Check sheet for the modelled part. Datum: model origin and axes. Units: mm. Face numbers are marked on the shaded views. A direction names the side the tool comes from. Round coordinates to 2 decimals unless told otherwise and drop trailing zeros. Write each loop counter-clockwise with the first axis right and the second up, starting at its lowest first coordinate (ties: lowest second). Pieces come first, ordered by that corner, then holes. Notation, with made-up numbers: (33.25, 46.25) -> (63.25, 46.25) arc R8 cw to (63.25, 52.25) -> close; hole circle Ø1 at (33, -17.5). An arc over 180 degrees is marked (long way). Write item = value, one per line.
from build123d import *

# Parameters (mm, degrees)
SKETCH1_W              = 165.1
SKETCH1_H              = 47.498
BOSS_EXTRUDE1_DEPTH    = 22.098
CUT_EXTRUDE1_DEPTH     = 18.249011
F_10_32_TAPPED_HOLE1_D = 4.0386


with BuildPart() as part:
    # Sketch1 → Boss-Extrude1 (new body)
    with BuildSketch(Plane(origin=(0, 0, 0), x_dir=(0, 0, -1), z_dir=(1, 0, 0))):
        Rectangle(SKETCH1_W, SKETCH1_H)
        with BuildLine():
            Line((-67.5752522, 2.5527), (67.5752522, 2.5527))
            ThreePointArc((67.5752522, 2.5527), (70.1279522, 0), (67.5752522, -2.5527))
            Line((67.5752522, -2.5527), (-67.5752522, -2.5527))
            ThreePointArc((-67.5752522, -2.5527), (-70.1279522, 0), (-67.5752522, 2.5527))
        make_face(mode=Mode.SUBTRACT)
    extrude(amount=BOSS_EXTRUDE1_DEPTH)

    # Sketch2 → Cut-Extrude1 (cut)
    with BuildSketch(Plane(origin=(22.098, 0, 0), x_dir=(0, 0, -1), z_dir=(1, 0, 0))):
        with BuildLine():
            Line((-67.5752522, 6.4797559), (67.5752522, 6.4797559))
            ThreePointArc((67.5752522, 6.4797559), (74.0550081, 0), (67.5752522, -6.4797559))
            Line((67.5752522, -6.4797559), (-67.5752522, -6.4797559))
            ThreePointArc((-67.5752522, -6.4797559), (-74.0550081, 0), (-67.5752522, 6.4797559))
        make_face()
    extrude(amount=-CUT_EXTRUDE1_DEPTH, mode=Mode.SUBTRACT)

    # #10-32 Tapped Hole1 (through all)
    with Locations(Plane(origin=(22.098, 0, 0), x_dir=(0, 0, -1), z_dir=(1, 0, 0))):
        with Locations((-76.2, 17.399), (-76.2, -17.399), (0, -17.399), (76.2, -17.399), (76.2, 17.399), (0, 17.399)):
            Hole(F_10_32_TAPPED_HOLE1_D / 2)


solid = part.part
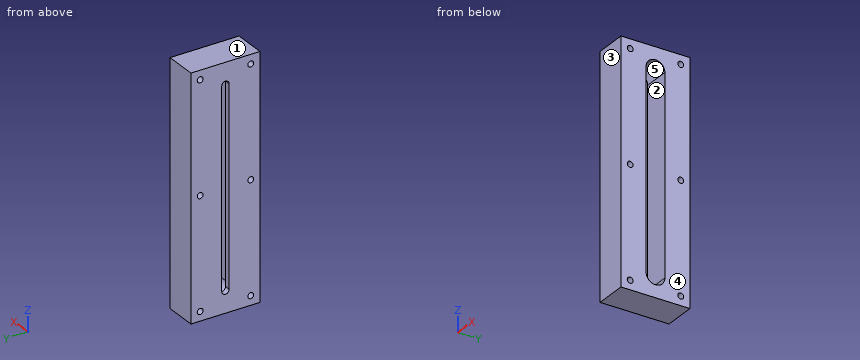
(1) Sectioned sample at C-C on y = 0.5. Enter the section's corners in (x, z).
Worked answers:
outline = (0, -82.55) -> (22.1, -82.55) -> (22.1, -74.04) -> (3.85, -74.04) -> (3.85, -70.08) -> (0, -70.08) -> close; (0, 70.08) -> (3.85, 70.08) -> (3.85, 74.04) -> (22.1, 74.04) -> (22.1, 82.55) -> (0, 82.55) -> close
(2) Sectioned sample at D-D on z = 76.2. Enter the section's corners in (x, y), then the cut area to 3 significant figures.
Worked answers:
outline = (0, -23.75) -> (22.1, -23.75) -> (22.1, -19.42) -> (0, -19.42) -> close; (0, -15.38) -> (22.1, -15.38) -> (22.1, 15.38) -> (0, 15.38) -> close; (0, 19.42) -> (22.1, 19.42) -> (22.1, 23.75) -> (0, 23.75) -> close
area = 871 mm²
(3) Sectioned sample at A-A on z = 0. Enter the section's corners in (x, y), then the cut area to 3 significant figures.
Worked answers:
outline = (0, -23.75) -> (22.1, -23.75) -> (22.1, -19.42) -> (0, -19.42) -> close; (0, -15.38) -> (22.1, -15.38) -> (22.1, -6.48) -> (3.85, -6.48) -> (3.85, -2.55) -> (0, -2.55) -> close; (0, 2.55) -> (3.85, 2.55) -> (3.85, 6.48) -> (22.1, 6.48) -> (22.1, 15.38) -> (0, 15.38) -> close; (0, 19.42) -> (22.1, 19.42) -> (22.1, 23.75) -> (0, 23.75) -> close
area = 615 mm²
(4) Go/stop test with flat-tipped pins: P1, Ø2.5, axis at y = -17.399, z = -76.2, coming from the +X side; P2, Ø6.5, axis at y = -1.5, z = -12, coming from the +X side. Record where each tip stops, or that it passes through.
Worked answers:
P1 = through
P2 = 3.85
(5) Sectioned sample at B-B on z = -48.5. Enter the section's corners in (x, y), then the cut area to 3 significant figures.
Worked answers:
outline = (0, -23.75) -> (22.1, -23.75) -> (22.1, -6.48) -> (3.85, -6.48) -> (3.85, -2.55) -> (0, -2.55) -> close; (0, 2.55) -> (3.85, 2.55) -> (3.85, 6.48) -> (22.1, 6.48) -> (22.1, 23.75) -> (0, 23.75) -> close
area = 793 mm²
(6) Access from +Z, -Z, +X, -X, +Y, -Y to the whole of each face (thin tool, end or side, straight path). Record for the marked faces 1 and 2.
Worked answers:
face_1 = +Z, +X, -X, +Y, -Y
face_2 = +X
(7) Material ranges on L1, parallel to Y at x = 7.5, z = 0; L2, parallel to Y at x = 12.5, z = -76.2; L3, parallel to Y at x = 14.25, z = -23.5, recorded low to high. Write a range as [from, to].
Worked answers:
L1 = [-23.75, -19.42], [-15.38, -6.48], [6.48, 15.38], [19.42, 23.75]
L2 = [-23.75, -19.42], [-15.38, 15.38], [19.42, 23.75]
L3 = [-23.75, -6.48], [6.48, 23.75]
(8) Release check for a two-part mould opening along Y. For the marked faces 3, 4 and 5 record: pulls with the +Y half, pulls with the -Y half, needs draft (parallel to the pull), parting line crosses it, or undercut.
Worked answers:
face_3 = pulls with the -Y half
face_4 = needs draft
face_5 = undercut
